The listing builds one solid part. Answer for the finished solid, in the listing's coordinates (mm). Coordinates: 2 decimals unless noted, no trailing zeros. Order: outer loops, then holes, each group sorted by start corner. A loop starts at its lowest first (then second) coordinate and runs counter-clockwise, first axis right, second up. Notation, with made-up numbers: (-25, 3) - (21, 3) arc R20 ccw to (21, 33) - close; hole circle Ø8 at (24, 66.25). An arc over 180 degrees is marked (long way). One line per item, written item: value. Start each with the question number.
```python
from build123d import *

# Parameters (mm, degrees)
MODEL_R             = 2
MODEL_W             = 27.5
MODEL_H             = 40
MODEL_W_2           = 100
MODEL_H_2           = 5
MODEL_H_3           = 3
EXTRUDE_1_DEPTH     = 3
SKETCH_2_R          = 2
CUT_EXTRUDE_1_DEPTH = 10


with BuildPart() as part:
    # Model → 凸台-拉伸1 (new body)
    with BuildSketch(Plane.XY):
        with BuildLine():
            Line((130, -77), (130, 77))
            ThreePointArc((130, 77), (129.121320344, 79.121320344), (127, 80))
            Line((127, 80), (-127, 80))
            ThreePointArc((-127, 80), (-129.121320344, 79.121320344), (-130, 77))
            Line((-130, 77), (-130, -77))
            ThreePointArc((-130, -77), (-129.121320344, -79.121320344), (-127, -80))
            Line((-127, -80), (127, -80))
            ThreePointArc((127, -80), (129.121320344, -79.121320344), (130, -77))
        make_face()
        with Locations((-110, 49)):
            Circle(MODEL_R, mode=Mode.SUBTRACT)
        with Locations((-80, 73)):
            Circle(MODEL_R, mode=Mode.SUBTRACT)
        with Locations((110, 73)):
            Circle(MODEL_R, mode=Mode.SUBTRACT)
        with Locations((-120, 73)):
            Circle(MODEL_R, mode=Mode.SUBTRACT)
        with Locations((80, 73)):
            Circle(MODEL_R, mode=Mode.SUBTRACT)
        with Locations((110, 49)):
            Circle(MODEL_R, mode=Mode.SUBTRACT)
        with Locations((80, -49)):
            Circle(MODEL_R, mode=Mode.SUBTRACT)
        with Locations((110, -73)):
            Circle(MODEL_R, mode=Mode.SUBTRACT)
        with Locations((-80, -73)):
            Circle(MODEL_R, mode=Mode.SUBTRACT)
        with Locations((-110, -49)):
            Circle(MODEL_R, mode=Mode.SUBTRACT)
        with Locations((-80, -49)):
            Circle(MODEL_R, mode=Mode.SUBTRACT)
        with Locations((-110, -73)):
            Circle(MODEL_R, mode=Mode.SUBTRACT)
        with Locations((80, -73)):
            Circle(MODEL_R, mode=Mode.SUBTRACT)
        with Locations((110, -49)):
            Circle(MODEL_R, mode=Mode.SUBTRACT)
        with Locations((80, 49)):
            Circle(MODEL_R, mode=Mode.SUBTRACT)
        with Locations((120, 73)):
            Circle(MODEL_R, mode=Mode.SUBTRACT)
        with Locations((120, -73)):
            Circle(MODEL_R, mode=Mode.SUBTRACT)
        with Locations((-110, 73)):
            Circle(MODEL_R, mode=Mode.SUBTRACT)
        with Locations((-80, 49)):
            Circle(MODEL_R, mode=Mode.SUBTRACT)
        with Locations((-120, -73)):
            Circle(MODEL_R, mode=Mode.SUBTRACT)
        with Locations((-101.25, 0)):
            Rectangle(MODEL_W, MODEL_H, mode=Mode.SUBTRACT)
        with Locations((101.25, 0)):
            Rectangle(MODEL_W, MODEL_H, mode=Mode.SUBTRACT)
        with Locations((0, -65)):
            Rectangle(MODEL_W_2, MODEL_H_2, mode=Mode.SUBTRACT)
        with Locations((0, 65)):
            Rectangle(MODEL_W_2, MODEL_H_2, mode=Mode.SUBTRACT)
        Rectangle(MODEL_W_2, MODEL_H_3, mode=Mode.SUBTRACT)
        with Locations((0, -40)):
            Rectangle(MODEL_W_2, MODEL_H_3, mode=Mode.SUBTRACT)
        with Locations((0, 40)):
            Rectangle(MODEL_W_2, MODEL_H_3, mode=Mode.SUBTRACT)
    extrude(amount=EXTRUDE_1_DEPTH)

    # 草图2 → 切除-拉伸1 (cut)
    with BuildSketch(Plane.XY.offset(3)):
        with Locations((-45, 30)):
            Circle(SKETCH_2_R)
        with Locations((45, 30)):
            Circle(SKETCH_2_R)
        with Locations((45, -30)):
            Circle(SKETCH_2_R)
        with Locations((-45, -30)):
            Circle(SKETCH_2_R)
    extrude(amount=-CUT_EXTRUDE_1_DEPTH, mode=Mode.SUBTRACT)


solid = part.part
```
(1) Flat-ended cylindrical pins translate along their axes: pin 1 Ø3 at (x, y) = (-110, 49) entering from -Z; pin 2 Ø5 at (x, y) = (-45, 30) entering from -Z. Find the tip coordinate at first contact, or state that the pin passes through.
(2) Consider probe 1 along Y at (x, z) = (3.5, 2.15); probe 2 along Y at (x, z) = (-120, 1.3); probe 3 along X at (y, z) = (-4.5, 0.35). Determine where each line is inside the solid, lowest interval first.
(3) The part is cut by section B-B on y = 13. Determine the outline of the cut face in (x, z), plus the area to 3 significant figures.
(4) The part is cut by section C-C on z = 0.95. Count the separate pieces of the cut face and the enclosed holes in it, plus the area to 3 significant figures.
(5) The part is cut by section A-A on x = 9.5. Determine the outline of the cut face in (y, z).
Completed:
1. pin 1: passes through
1. pin 2: stops at z = 0
2. probe 1: y = -80 to -67.5, -62.5 to -41.5, -38.5 to -1.5, 1.5 to 38.5, 41.5 to 62.5, 67.5 to 80
2. probe 2: y = -80 to -75, -71 to 71, 75 to 80
2. probe 3: x = -130 to -115, -87.5 to 87.5, 115 to 130
3. outline: (-130, 0) - (-115, 0) - (-115, 3) - (-130, 3) - close; (-87.5, 0) - (87.5, 0) - (87.5, 3) - (-87.5, 3) - close; (115, 0) - (130, 0) - (130, 3) - (115, 3) - close
3. area: 615 mm2
4. separate pieces: 1
4. enclosed holes: 31
4. area: 37,200 mm2
5. outline: (-80, 0) - (-67.5, 0) - (-67.5, 3) - (-80, 3) - close; (-62.5, 0) - (-41.5, 0) - (-41.5, 3) - (-62.5, 3) - close; (-38.5, 0) - (-1.5, 0) - (-1.5, 3) - (-38.5, 3) - close; (1.5, 0) - (38.5, 0) - (38.5, 3) - (1.5, 3) - close; (41.5, 0) - (62.5, 0) - (62.5, 3) - (41.5, 3) - close; (67.5, 0) - (80, 0) - (80, 3) - (67.5, 3) - close
